from build123d import *

# Parameters (mm, degrees)
F0_W     = 1000
F0_H     = 1000
F1_DEPTH = 1000
F2_R     = 50
F3_T     = -5
F4_R     = 125
F5_DEPTH = 650


# Not quite as in the source:
# - a shell that OpenCascade refuses in one call is made with other operations: the cavity is built on its own and cut out


with BuildPart() as f1:
    # F0 (on Top) → F1 (new body)
    with BuildSketch(Plane.XY):
        Rectangle(F0_W, F0_H)
    extrude(amount=F1_DEPTH)

    # F2
    f2_edges = [f1.edges().sort_by_distance(p)[0] for p in [
        (0, 500, 1000),
        (-500, 500, 500),
        (-500, 0, 1000),
        (500, 0, 1000),
        (500, 500, 500),
        (0, -500, 1000),
        (-500, -500, 500),
        (500, -500, 500),
        (500, 0, 0),
        (0, -500, 0),
        (0, 500, 0),
        (-500, 0, 0),
    ]]
    fillet(f2_edges, radius=F2_R)

    # F3: a shell. OpenCascade refuses it in one call, so the cavity is built on its own and cut out:
    # the body offset inwards by the wall thickness, plus a prism from it out through each open face.
    f3_core = offset(f1.part, amount=F3_T, mode=Mode.PRIVATE)
    f3_exits = [f3_core.faces().sort_by_distance(p)[0] for p in [
        (0, -495, 500),
    ]]
    add(f3_core, mode=Mode.SUBTRACT)
    extrude(f3_exits, amount=-F3_T, mode=Mode.SUBTRACT)

    # F4 (on Right) → F5 (cut, symmetric)
    with BuildSketch(Plane.YZ):
        with Locations((0, 300)):
            Circle(F4_R)
    extrude(amount=F5_DEPTH, both=True, mode=Mode.SUBTRACT)


solid = f1.part
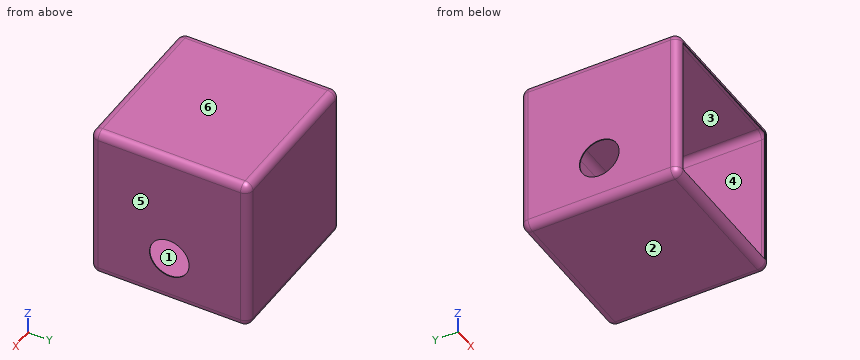
Check sheet for the modelled part. Datum: model origin and axes. Units: mm. Face numbers are marked on the shaded views. A direction names the side the tool comes from. Give positions to 0.01 mm unless a question says otherwise; leave off trailing zeros. Write each loop counter-clockwise with the first axis right and the second up, starting at its lowest first coordinate (ties: lowest second). Pieces come first, ordered by that corner, then holes. Notation, with made-up numbers: (-26, 69) -> (-12, 69) arc R22 ccw to (-12, 99) -> close; hole circle Ø5 at (6.25, 70). An arc over 180 degrees is marked (long way). Use one line per item in the form item = value. Start each with the question number.
1. Mould release check, pull along Z, two halves, no side actions. Record for the marked faces 3, 4, 5 and 6: pulls with the +Z half, pulls with the -Z half, needs draft (parallel to the pull), parting line crosses it, or undercut.
2. Section check C-C (x = -290.5). Record the cut outline in (y, z).
3. Section check D-D (y = 210). Record the cut outline in (x, z).
4. Go/stop test with flat-tipped pins: P1, Ø4, axis at x = -126.5, y = -498, coming from the -Z side; P2, Ø5.5, axis at x = 137.5, y = -496.5, coming from the +Z side; P3, Ø5.5, axis at y = -497.5, z = 723, coming from the +X side. Record where each tip stops, or that it passes through.
5. Section check A-A (y = 0). Record the cut outline in (x, z), and give its area (3 significant figures).
6. Section check B-B (z = 300). Record the cut outline in (x, y), and give its area (3 significant figures).
7. Thickness scan on line 1 along X through (y, z) = (-231, 404); line 2 along Z through (x, y) = (163.5, 26.5); line 3 along Y through (x, z) = (140, 880). Record the ranges inside material, lowest first. Write a range as from..to.
8. Access from +Z, -Z, +X, -X, +Y, -Y to the whole of each face (thin tool, end or side, straight path). Record for the marked faces 1 and 2.
Conclusion:
q1.face_3 = undercut
q1.face_4 = undercut
q1.face_5 = needs draft
q1.face_6 = pulls with the +Z half
q2.outline = (-500, 50) arc R50 ccw to (-450, 0) -> (450, 0) arc R50 ccw to (500, 50) -> (500, 950) arc R50 ccw to (450, 1000) -> (-450, 1000) arc R50 ccw to (-500, 950) -> (-495, 950) arc R45 cw to (-450, 995) -> (450, 995) arc R45 cw to (495, 950) -> (495, 50) arc R45 cw to (450, 5) -> (-450, 5) arc R45 cw to (-495, 50) -> close
q3.outline = (-500, 50) arc R50 ccw to (-450, 0) -> (450, 0) arc R50 ccw to (500, 50) -> (500, 950) arc R50 ccw to (450, 1000) -> (-450, 1000) arc R50 ccw to (-500, 950) -> close; hole (-495, 50) arc R45 ccw to (-450, 5) -> (450, 5) arc R45 ccw to (495, 50) -> (495, 950) arc R45 ccw to (450, 995) -> (-450, 995) arc R45 ccw to (-495, 950) -> close
q4.P1 = 30.4
q4.P2 = 974.21
q4.P3 = 472.3
q5.outline = (-500, 50) arc R50 ccw to (-450, 0) -> (450, 0) arc R50 ccw to (500, 50) -> (500, 175) -> (495, 175) -> (495, 50) arc R45 cw to (450, 5) -> (-450, 5) arc R45 cw to (-495, 50) -> (-495, 175) -> (-500, 175) -> close; (-500, 425) -> (-495, 425) -> (-495, 950) arc R45 cw to (-450, 995) -> (450, 995) arc R45 cw to (495, 950) -> (495, 425) -> (500, 425) -> (500, 950) arc R50 ccw to (450, 1000) -> (-450, 1000) arc R50 ccw to (-500, 950) -> close
q5.area = 17,000 mm²
q6.outline = (-500, -450) arc R50 ccw to (-450, -500) -> (-450, -495) arc R45 cw to (-495, -450) -> (-495, -125) -> (-500, -125) -> close; (-500, 125) -> (-495, 125) -> (-495, 450) arc R45 cw to (-450, 495) -> (450, 495) arc R45 cw to (495, 450) -> (495, 125) -> (500, 125) -> (500, 450) arc R50 ccw to (450, 500) -> (-450, 500) arc R50 ccw to (-500, 450) -> close; (450, -500) arc R50 ccw to (500, -450) -> (500, -125) -> (495, -125) -> (495, -450) arc R45 cw to (450, -495) -> close
q6.area = 12,500 mm²
q7.line_1 = -500..-495, 495..500
q7.line_2 = 0..5, 995..1000
q7.line_3 = 495..500
q8.face_1 = none
q8.face_2 = -Z, +X, -X, +Y, -Y
